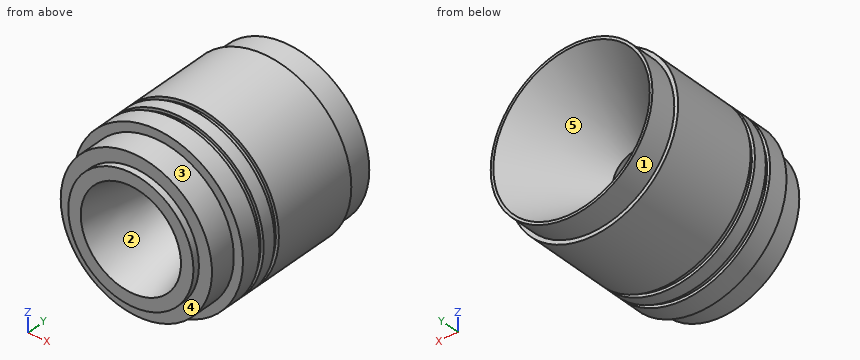
from build123d import *

# Parameters (mm, degrees)
SZKIC2_W = 2.3
SZKIC2_H = 3.9


with BuildPart() as part:
    # Szkic1 → Obrót1 (revolve)
    with BuildSketch(Plane.XY, mode=Mode.PRIVATE) as obr_t1_sk:
        Polygon((60, 64.358983849), (18.436392049, 5), (18.436392049, -5), (38.436392049, -79.641016151), (48, -79.641016151), (48, -74.641016151), (58, -74.641016151), (58, -54.641016151), (65, -54.641016151), (65, 44.358983849), (62, 44.358983849), (62, 64.358983849), align=None)
    revolve(obr_t1_sk.sketch.rotate(Axis((0, 60.824555965, 0), (0, -1, 0)), 180), axis=Axis((0, 60.824555965, 0), (0, -1, 0)))

    # Szkic2 → Wycięcie-obrót1 (revolve, cut)
    with BuildSketch(Plane.XY, mode=Mode.PRIVATE) as wyci_cie_obr_t1_sk:
        with Locations((63.85, -37.691016151)):
            Rectangle(SZKIC2_W, SZKIC2_H)
        with Locations((63.85, -23.791016151)):
            Rectangle(SZKIC2_W, SZKIC2_H)
    revolve(wyci_cie_obr_t1_sk.sketch.rotate(Axis((0, 85.874550226, 0), (0, -1, 0)), 90), axis=Axis((0, 85.874550226, 0), (0, -1, 0)), mode=Mode.SUBTRACT)


solid = part.part
Geometry: final body of the model. Coordinates: model frame, mm. Face numbers are marked on the shaded views. A direction names the side the tool comes from. Coordinates: 2 decimals unless noted, no trailing zeros. Loops run counter-clockwise (first coordinate to the right, second up) from the corner with the lowest first, then second, coordinate; pieces in that order, holes last. Notation, with made-up numbers: (11.5, 73) - (52.5, 73) arc R32 ccw to (52.5, 103) - close; hole circle Ø5 at (-26.5, -27). An arc over 180 degrees is marked (long way). Put each result on its own line as item: value. Start each with the question number.
Q1. Pin query (flat end, axial travel): pin 1 Ø12 at (x, z) = (12, 47.5) entering from -Y; pin 2 Ø10 at (y, z) = (-18, -19.5) entering from +X; pin 3 Ø22 at (x, z) = (0, 0) entering from +Y; pin 4 Ø6 at (y, z) = (-57, -15) entering from -X. Return the tip coordinate at first contact, or that it passes through.
Q2. Pull-direction query (Z, two-part tool) for the marked faces 3, 4 and 5; classes: released by +Z, released by -Z, zero draft, split by the parting line, or undercut.
Q3. Line query: line 1 (Y direction, x = 37.5, z = -52); line 2 (X direction, y = 5, z = 1); line 3 (Z direction, x = 0, y = 2). Output: solid intervals per line, ascending.
Q4. Set-up query: the marked faces 1 and 2. Return all of +Z, -Z, +X, -X, +Y, -Y with unobstructed straight access to the full face (end or side cutting, diameter ignored); none if empty.
Q5. Cut plane B-B, the plane y = -7. Return loops of the section in (x, z), and give its area (3 significant figures).
Q6. Cut plane A-A, the plane y = -65. Return loops of the section in (x, z), and give its area (3 significant figures).
Filled sheet:
1. pin 1: y = -79.64
1. pin 2: x = 63.36
1. pin 3: through
1. pin 4: x = -63.66
2. face 3: split by the parting line
2. face 4: zero draft
2. face 5: undercut
3. line 1: -54.64 to -39.64, -35.74 to -25.74, -21.84 to 44.36
3. line 2: -64.99 to -18.41, 18.41 to 64.99
3. line 3: -65 to -18.44, 18.44 to 65
4. face 1: +Y
4. face 2: -Y
5. outline: circle Ø130 at (0, 0); hole circle Ø37.94 at (0, 0)
5. area: 12,100 mm²
6. outline: circle Ø116 at (0, 0); hole circle Ø69.03 at (0, 0)
6. area: 6,830 mm²
